The listing builds one solid part. Answer for the finished solid, in the listing's coordinates (mm). Face numbers are marked on the shaded views. Round coordinates to 2 decimals unless told otherwise and drop trailing zeros. Write item = value, one per line. Start each with the question number.
(1) Each of these flat-tipped pins is pushed along its axis until it touches: pin 1 (1.5 mm diameter, centred on x = -1.5, z = 2.5, fed in from -Y); pin 2 (1.8 mm diameter, centred on x = 0, y = -0.01, fed in from +Z); pin 3 (3 mm diameter, centred on y = -2, z = 2, fed in from -X) (3 decimals). Where does it stop, or does it pass through?
(2) Straight lines are drawn through the part: probe 1 along Z at (x, y) = (-1.25, -0.5); probe 2 along Y at (x, z) = (1, 2.5); probe 3 along X at (y, z) = (-1.25, 5.75). For each, find the intervals that lie inside material, in ascending order. Write a range as from..to.
(3) For a pull along Y with two mould halves and no side action, classify the marked faces 1 and 2 as released by +Y, released by -Y, zero draft, split by the parting line, or undercut.
from build123d import *

# Parameters (mm, degrees)
F0_R     = 2.5
F0_R_2   = 1.5
F1_DEPTH = 6
F2_R     = 2.5
F3_R     = 4
F5_R     = 1.5
F6_DEPTH = 4


with BuildPart() as f1:
    # F0 (on Top) → F1 (new body)
    with BuildSketch(Plane.XY):
        Circle(F0_R)
        Circle(F0_R_2, mode=Mode.SUBTRACT)
    extrude(amount=F1_DEPTH)

    # F2 (on face) → F4 section 0
    with BuildSketch(Plane.XY.offset(6)):
        Circle(F2_R)
    # F3 (on face) → F4 section 1
    with BuildSketch(Plane.XY):
        with Locations((0.01406, 0.042179)):
            Circle(F3_R)
    loft()

    # F5 (on face) → F6 (cut)
    with BuildSketch(Plane.XY.offset(6)):
        with Locations((0.001315, -0.013137)):
            Circle(F5_R)
    extrude(amount=-F6_DEPTH, mode=Mode.SUBTRACT)


solid = f1.part
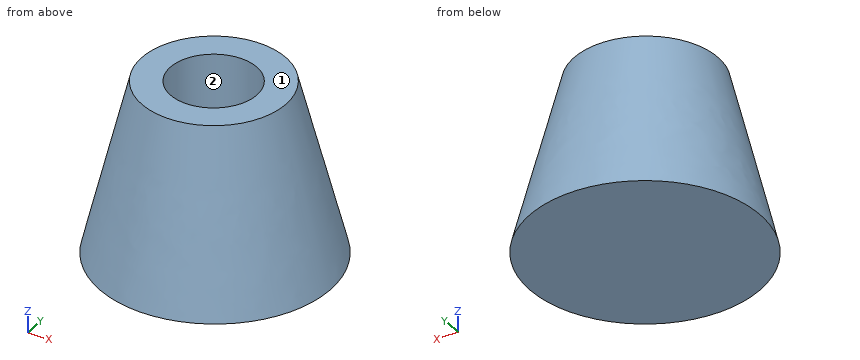
Reported:
q1.pin_1 = -3.34
q1.pin_2 = 2
q1.pin_3 = -3.625
q2.probe_1 = 0..2
q2.probe_2 = -3.2..-1.13, 1.11..3.25
q2.probe_3 = -2.24..-0.85, 0.85..2.24
q3.face_1 = zero draft
q3.face_2 = undercut
